Build history of the part. All positions in model axes, mm. Face numbers are marked on the shaded views. A direction names the side the tool comes from. Round coordinates to 2 decimals unless told otherwise and drop trailing zeros. Loops run counter-clockwise (first coordinate to the right, second up) from the corner with the lowest first, then second, coordinate; pieces in that order, holes last. Notation, with made-up numbers: (51.25, -33) - (71.25, -33) arc R27 cw to (71.25, -13) - close; hole circle Ø8 at (1, 45). An arc over 180 degrees is marked (long way). Put each result on its own line as item: value. Start each with the question number.
from build123d import *

# Parameters (mm, degrees)
PAD_DEPTH           = 120
SKETCH_R            = 1.55
PAD001_DEPTH        = 20
LINEARPATTERN_COUNT = 2
LINEARPATTERN_PITCH = 74
SKETCH002_W         = 25
SKETCH002_H         = 30
POCKET_DEPTH        = 120.001
SKETCH003_R         = 1.6
POCKET001_DEPTH     = 13.001
SKETCH004_R         = 1.6
POCKET002_DEPTH     = 13
SKETCH005_R         = 1.6
POCKET003_DEPTH     = 93.001
SKETCH006_R         = 1.55
PAD002_DEPTH        = 26
POCKET004_DEPTH     = 13.001
FILLET_R            = 3
FILLET_FACE44_R     = 1.55
PAD003_DEPTH        = 6.5
SKETCH008_R         = 6.4
POCKET005_DEPTH     = 3
SKETCH009_R         = 1.5
POCKET006_DEPTH     = 5
SKETCH010_W         = 25.4
SKETCH010_H         = 112.9
POCKET007_DEPTH     = 1.2
FILLET001_R         = 3.5


with BuildPart() as body001:
    # Sketch001 → Pad (new body)
    with BuildSketch(Plane.XZ):
        Polygon((-70, 45), (-32.1173210497, 45), (-0.1173210497, -45), (50, -45), (50, -42), (2, -42), (-30, 48), (-70, 48), align=None)
    extrude(amount=PAD_DEPTH)

    # Sketch (on Face10 of Pad) → Pad001 (join)
    with BuildSketch(Plane.XZ.offset(120)):
        Polygon((50, -45), (50, -32), (-4.7395432719, -32), (-0.1173210497, -45), align=None)
        with Locations((10.2, -37)):
            Circle(SKETCH_R, mode=Mode.SUBTRACT)
        with Locations((41.8, -37)):
            Circle(SKETCH_R, mode=Mode.SUBTRACT)
    pad001 = extrude(amount=-PAD001_DEPTH)

    # LinearPattern: Pad001 ×2
    with Locations(*[(0, i * LINEARPATTERN_PITCH, 0) for i in range(1, LINEARPATTERN_COUNT)]):
        add(pad001)

    # Sketch002 (on Face2 of LinearPattern) → Pocket (cut, through all)
    with BuildSketch(Plane(origin=(-70, 0, 0), x_dir=(0, 0, -1), z_dir=(-1, 0, 0))):
        with Locations((-35.5, 105)):
            Rectangle(SKETCH002_W, SKETCH002_H)
    extrude(amount=-POCKET_DEPTH, mode=Mode.SUBTRACT)

    # Sketch003 (on Face18 of Pocket) → Pocket001 (cut, through all)
    with BuildSketch(Plane(origin=(0, 0, -32), x_dir=(-1, 0, 0), z_dir=(0, 0, 1))):
        with Locations((-37.6, 110)):
            Circle(SKETCH003_R)
        with Locations((-14.4, 110)):
            Circle(SKETCH003_R)
    extrude(amount=-POCKET001_DEPTH, mode=Mode.SUBTRACT)

    # Sketch004 (on Face16 of Pocket001) → Pocket002 (cut)
    with BuildSketch(Plane(origin=(0, 0, -32), x_dir=(-1, 0, 0), z_dir=(0, 0, 1))):
        with Locations((-40, 13)):
            Circle(SKETCH004_R)
        with Locations((-40, 86.5)):
            Circle(SKETCH004_R)
        with Locations((-40, 59.5)):
            Circle(SKETCH004_R)
    extrude(amount=-POCKET002_DEPTH, mode=Mode.SUBTRACT)

    # Sketch005 (on Face10 of Pocket002) → Pocket003 (cut, through all)
    with BuildSketch(Plane(origin=(0, 0, 48), x_dir=(-1, 0, 0), z_dir=(0, 0, 1))):
        with Locations((60, 56.25)):
            Circle(SKETCH005_R)
        with Locations((60, 33.75)):
            Circle(SKETCH005_R)
        with Locations((60, 78.75)):
            Circle(SKETCH005_R)
        with Locations((60, 11.25)):
            Circle(SKETCH005_R)
    extrude(amount=-POCKET003_DEPTH, mode=Mode.SUBTRACT)

    # Sketch006 (on Face16 of Pocket003) → Pad002 (join)
    with BuildSketch(Plane.XZ.offset(120)):
        Polygon((-4.7395432719, -32), (-0.1173210497, -45), (50, -45), (50, -32), align=None)
        with Locations((10.2, -37)):
            Circle(SKETCH006_R, mode=Mode.SUBTRACT)
        with Locations((41.8, -37)):
            Circle(SKETCH006_R, mode=Mode.SUBTRACT)
    extrude(amount=PAD002_DEPTH)

    # Sketch007 (on Face30 of Pad002) → Pocket004 (cut, through all)
    with BuildSketch(Plane(origin=(0, 0, -32), x_dir=(-1, 0, 0), z_dir=(0, 0, 1))):
        with BuildLine():
            ThreePointArc((-37, 141), (-45, 133), (-37, 125))
            Line((-37, 125), (-8.2604567281, 125))
            ThreePointArc((-8.2604567281, 125), (-0.2604567281, 133), (-8.2604567281, 141))
            Line((-37, 141), (-8.2604567281, 141))
        make_face()
    extrude(amount=-POCKET004_DEPTH, mode=Mode.SUBTRACT)

    # Fillet
    fillet_edges = [body001.edges().sort_by_distance(p)[0] for p in [
        (-70, -90, 46.5),
        (-22.703105, -90, 23),
        (-22.703105, -120, 23),
        (-2.428432, -146, -38.5),
        (-3.147549, -120, -32),
        (50, -146, -38.5),
        (2, -73, -42),
        (2, -13, -42),
        (-30, -45, 48),
        (-32.117321, -45, 45),
        (-0.117321, -73, -45),
    ]]
    fillet(fillet_edges, radius=FILLET_R)

    # Fillet Face44 → Pad003 (add)
    with BuildSketch(Plane(origin=(25.1111807408, -100, -36.9307209513), x_dir=(1, 0, 0), z_dir=(0, 1, 0))):
        with BuildLine():
            Line((-23.8205037619, 3.0743080517), (-26.6667362963, -4.9307209513))
            Line((-26.6667362963, -4.9307209513), (24.8888192592, -4.9307209513))
            Line((24.8888192592, -4.9307209513), (24.8888192592, 5.0692790487))
            Line((24.8888192592, 5.0692790487), (-20.9938596911, 5.0692790487))
            ThreePointArc((-20.9938596911, 5.0692790487), (-22.7237315059, 4.5203081192), (-23.8205037619, 3.0743080517))
        make_face()
        with Locations((-14.9111807408, 0.0692790487)):
            Circle(FILLET_FACE44_R, mode=Mode.SUBTRACT)
        with Locations((16.6888192592, 0.0692790487)):
            Circle(FILLET_FACE44_R, mode=Mode.SUBTRACT)
    extrude(amount=PAD003_DEPTH)

    # Sketch008 (on Face12 of Pad003) → Pocket005 (cut)
    with BuildSketch(Plane(origin=(0, 0, 48), x_dir=(-1, 0, 0), z_dir=(0, 0, 1))):
        with Locations((41, 65)):
            Circle(SKETCH008_R)
    extrude(amount=-POCKET005_DEPTH, mode=Mode.SUBTRACT)

    # Sketch009 (on Face12 of Pocket005) → Pocket006 (cut)
    with BuildSketch(Plane(origin=(-14.3084502962, 0, -5.0874489942), x_dir=(0.3350096677, 0, -0.9422146903), z_dir=(-0.9422146903, 0, -0.3350096677))):
        with Locations((-25.756963673, 54)):
            Circle(SKETCH009_R)
        with Locations((35.243036327, 54)):
            Circle(SKETCH009_R)
        with Locations((24.243036327, 54)):
            Circle(SKETCH009_R)
        with Locations((-14.756963673, 54)):
            Circle(SKETCH009_R)
        with Locations((-14.756963673, 11)):
            Circle(SKETCH009_R)
        with Locations((24.243036327, 11)):
            Circle(SKETCH009_R)
        with Locations((35.243036327, 11)):
            Circle(SKETCH009_R)
        with Locations((-25.756963673, 11)):
            Circle(SKETCH009_R)
        with Locations((-2.256963673, 54)):
            Circle(SKETCH009_R)
        with Locations((11.743036327, 54)):
            Circle(SKETCH009_R)
    extrude(amount=-POCKET006_DEPTH, mode=Mode.SUBTRACT)

    # Sketch010 (on Face13 of Pocket006) → Pocket007 (cut)
    with BuildSketch(Plane(origin=(0, 0, 48), x_dir=(-1, 0, 0), z_dir=(0, 0, 1))):
        with Locations((41.3, 0)):
            Rectangle(SKETCH010_W, SKETCH010_H)
    extrude(amount=-POCKET007_DEPTH, mode=Mode.SUBTRACT)

    # Fillet001
    fillet001_edges = [body001.edges().sort_by_distance(p)[0] for p in [
        (-54, -56.45, 47.4),
    ]]
    fillet(fillet001_edges, radius=FILLET001_R)


with BuildPart() as part_mirroring:
    # Part__Mirroring: instance of Body001
    add(body001.part.mirror(Plane(origin=(0, 0, 0), x_dir=(1, 0, 0), z_dir=(0, 1, 0))))


solid = part_mirroring.part
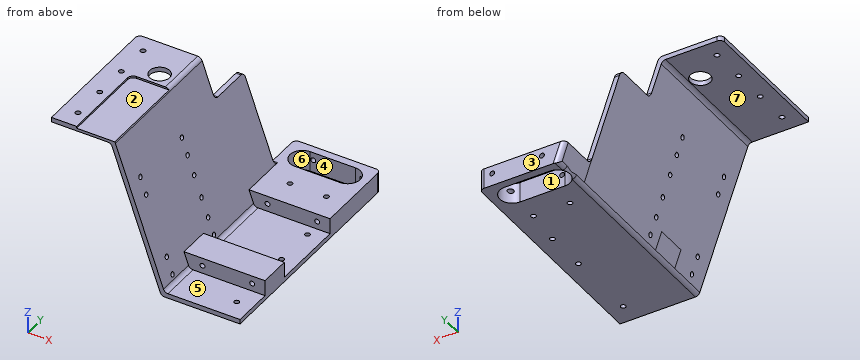
Item 1: Two-plate mould, pull along Y, no slides. Class the marked faces 1, 2, 3 and 4: pulls with the +Y half, pulls with the -Y half, needs draft (parallel to the pull), parting line crosses it, or undercut.
Item 2: Which spindle directions (+Z, -Z, +X, -X, +Y, -Y) get a long thin tool onto all of the face, cutting with end or side? Do the marked faces 5, 6 and 7. Say none if no direction does.
Item 3: Drill centre lines: probe 1 along X at (y, z) = (115, -37); probe 2 along Y at (x, z) = (37, -36); probe 3 along Z at (x, y) = (-55, 51.5). Where is each one in solid material? Low to high. Write a range as [from, to].
Item 4: Slice it at A-A (y = 43.5). Give the cut face in (x, z).
Item 5: Slice it at C-C (y = 82.5). Give the cut face in (x, z), plus the area to 3 significant figures.
Item 6: Slice it at B-B (x = -41). Give the cut face in (y, z), plus the area to 3 significant figures.
Item 7: Drop flat-ended pins along their axis: pin 1 Ø1 at (x, y) = (16, 56.5) entering from +Z; pin 2 Ø12 at (x, z) = (-35.5, 24.5) entering from -Y; pin 3 Ø12 at (y, z) = (90.5, 0.5) entering from -X; pin 4 Ø0.6 at (x, z) = (-42.5, 47.5) entering from -Y. Give the stop position or say it passes through.
Item 8: Slice it at D-D (x = 20). Give the cut face in (y, z), plus the area to 3 significant figures.
Computed values:
1. face 1: undercut
1. face 2: needs draft
1. face 3: pulls with the +Y half
1. face 4: undercut
2. face 5: +Z, +X, -Y
2. face 6: +Z, -Z
2. face 7: -Z, -X, +Y, -Y
3. probe 1: x = [-2.96, 8.65], [11.75, 40.25], [43.35, 50]
3. probe 2: y = [26, 46], [93.5, 108.52], [111.48, 125], [141, 146]
3. probe 3: z = [45, 48]
4. outline: (-70, 45) - (-34.23, 45) arc R3 cw to (-31.41, 43.01) - (-0.83, -43.01) arc R3 ccw to (2, -45) - (50, -45) - (50, -32) - (-1.56, -32) - (-29.29, 46.01) arc R3 ccw to (-29.72, 46.8) - (-54, 46.8) - (-54, 48) - (-70, 48) - close; hole circle Ø3.1 at (10.2, -37); hole circle Ø3.1 at (41.8, -37)
5. outline: (-70, 45) - (-34.23, 45) arc R3 cw to (-31.41, 43.01) - (-0.83, -43.01) arc R3 ccw to (2, -45) - (50, -45) - (50, -42) - (4.12, -42) arc R3 cw to (1.29, -40.01) - (-29.29, 46.01) arc R3 ccw to (-32.12, 48) - (-70, 48) - close
5. area: 551 mm^2
6. outline: (0, 45) - (58.6, 45) - (58.6, 48) - (56.45, 48) - (56.45, 46.8) - (0, 46.8) - close; (71.4, 45) - (90, 45) - (90, 48) - (71.4, 48) - close
6. area: 164 mm^2
7. pin 1: stops at z = -42
7. pin 2: passes through
7. pin 3: stops at x = -18.43
7. pin 4: stops at y = 56.45
8. outline: (0, -45) - (125, -45) - (125, -32) - (93.5, -32) - (93.5, -42) - (46, -42) - (46, -32) - (26, -32) - (26, -42) - (0, -42) - close; (141, -45) - (146, -45) - (146, -32) - (141, -32) - close
8. area: 955 mm^2
